Geometry check sheet. Reference: the model listing, model coordinates, mm. A direction names the side the tool comes from. Give positions to 0.01 mm unless a question says otherwise; leave off trailing zeros. Loops run counter-clockwise (first coordinate to the right, second up) from the corner with the lowest first, then second, coordinate; pieces in that order, holes last. Notation, with made-up numbers: (77, 43.25) -> (120, 43.25) arc R16 ccw to (120, 47.25) -> close; hole circle Ø2 at (5, 39). An arc over 180 degrees is marked (long way). One line per question, with ' | ' between items.
from build123d import *

# Parameters (mm, degrees)
IZIM1_R                     = 30
Y_KSEKLIK_EKSTR_ZYON1_DEPTH = 50
SCALE1_SCALE                = 0.5
SKETCH2_R                   = 12.5
CUT_EXTRUDE1_DEPTH          = 5
CUT_EXTRUDE2_START          = -10
SKETCH3_R                   = 12.5
CUT_EXTRUDE2_DEPTH          = 10
SKETCH4_R                   = 1
CUT_EXTRUDE3_DEPTH          = 10


with BuildPart() as part:
    # Çizim1 → Yükseklik-Ekstrüzyon1 (new body)
    with BuildSketch(Plane.XY):
        with Locations((-8.148787303, -1.554097453)):
            Circle(IZIM1_R)
    extrude(amount=Y_KSEKLIK_EKSTR_ZYON1_DEPTH)


with BuildPart() as part_1:
    # Scale1: scaled about (-8.148787303, -1.554097453, 25)
    add(part.part.scale(SCALE1_SCALE).moved(Location((-4.074393652, -0.777048727, 12.5))))

    # Sketch2 → Cut-Extrude1 (cut)
    with BuildSketch(Plane(origin=(0, 0, 12.5), x_dir=(-1, 0, 0), z_dir=(0, 0, -1))):
        with Locations((8.148787303, -1.554097453)):
            Circle(SKETCH2_R)
    extrude(amount=-CUT_EXTRUDE1_DEPTH, mode=Mode.SUBTRACT)

    # Sketch3 → Cut-Extrude2 (cut)
    with BuildSketch(Plane.XY.offset(37.5).offset(CUT_EXTRUDE2_START)):
        with Locations(Location((-8.148787303, -1.554097453, 0), (0, 0, 180))):
            Circle(SKETCH3_R)
    extrude(amount=CUT_EXTRUDE2_DEPTH, mode=Mode.SUBTRACT)

    # Sketch4 → Cut-Extrude3 (cut)
    with BuildSketch(Plane(origin=(0, 0, 17.5), x_dir=(-1, 0, 0), z_dir=(0, 0, -1))):
        with Locations((15.566518124, -5.706210793)):
            Circle(SKETCH4_R)
        with Locations((0.84408626, -5.901984113)):
            Circle(SKETCH4_R)
        with Locations((8.035757524, 6.945902547)):
            Circle(SKETCH4_R)
    extrude(amount=-CUT_EXTRUDE3_DEPTH, mode=Mode.SUBTRACT)


solid = part_1.part
Item 1: Scan lines: probe 1 along Z at (x, y) = (-6.75, -13.25); probe 2 along X at (y, z) = (-4.25, 30.75); probe 3 along Y at (x, z) = (-18, 30). Record each from-to range of solid material in increasing order.
Result:
probe 1: 17.5 to 27.5 | probe 2: -22.9 to -20.35, 4.06 to 6.61 | probe 3: -12.87 to -9.25, 6.14 to 9.76
Item 2: Sectioned sample at B-B (x = -15.25). Record the cut outline in (y, z), plus the area to 3 significant figures.
Result:
outline: (-14.77, 12.5) -> (-11.84, 12.5) -> (-11.84, 17.5) -> (-6.65, 17.5) -> (-6.65, 27.5) -> (-11.84, 27.5) -> (-11.84, 37.5) -> (-14.77, 37.5) -> close; (-4.76, 17.5) -> (8.73, 17.5) -> (8.73, 12.5) -> (11.66, 12.5) -> (11.66, 37.5) -> (8.73, 37.5) -> (8.73, 27.5) -> (-4.76, 27.5) -> close | area: 333 mm2
Item 3: Sectioned sample at D-D (y = -13.5). Record the cut outline in (x, z), plus the area to 3 significant figures.
Result:
outline: (-17.22, 12.5) -> (-11.83, 12.5) -> (-11.83, 17.5) -> (-4.47, 17.5) -> (-4.47, 12.5) -> (0.92, 12.5) -> (0.92, 37.5) -> (-4.47, 37.5) -> (-4.47, 27.5) -> (-11.83, 27.5) -> (-11.83, 37.5) -> (-17.22, 37.5) -> close | area: 343 mm2
Item 4: Sectioned sample at A-A (y = 7.5). Record the cut outline in (x, z), plus the area to 3 significant figures.
Result:
outline: (-20.11, 12.5) -> (-16.77, 12.5) -> (-16.77, 17.5) -> (-8.87, 17.5) -> (-8.87, 27.5) -> (-16.77, 27.5) -> (-16.77, 37.5) -> (-20.11, 37.5) -> close; (-7.2, 17.5) -> (0.47, 17.5) -> (0.47, 12.5) -> (3.81, 12.5) -> (3.81, 37.5) -> (0.47, 37.5) -> (0.47, 27.5) -> (-7.2, 27.5) -> close | area: 323 mm2
Item 5: Depth check by flat-ended pin: pin 1 Ø1.5 at (x, z) = (-17, 22) entering from +Y; pin 2 Ø3 at (y, z) = (9, 25) entering from +X; pin 3 Ø1 at (x, z) = (-7.5, 28.5) entering from -Y; pin 4 Ø2.5 at (x, y) = (-8.04, 6.95) entering from +Z. Enter the tip coordinate at first touch or a pass-through.
Result:
pin 1: y = 11.07 | pin 2: x = 3.81 | pin 3: y = -16.55 | pin 4: z = 27.5
Item 6: Release check for a two-part mould opening along Y. For faces 1 (the face through (-14, 10, 37.5)), 2 (the face through (-11.4, -16.197, 24.825)), 3 (the face through (0.155, -5.858, 22.43)) record: pulls with the +Y half, pulls with the -Y half, needs draft (parallel to the pull), parting line crosses it, or undercut.
Result:
face 1: needs draft | face 2: parting line crosses it | face 3: undercut
Item 7: Set-up check for faces 4 (the face through (-8, -2, 27.5)), 5 (the face through (-8, -1, 17.5)), 6 (the face through (-8.5, 6.06, 22.43)): record each of +Z, -Z, +X, -X, +Y, -Y from which the full face is reachable in a straight line by a thin tool's end or side.
Result:
face 4: +Z | face 5: -Z | face 6: +Z, -Z
Item 8: Sectioned sample at C-C (x = -6.5). Record the cut outline in (y, z), plus the area to 3 significant figures.
Result:
outline: (-16.46, 12.5) -> (-13.94, 12.5) -> (-13.94, 17.5) -> (10.84, 17.5) -> (10.84, 12.5) -> (13.36, 12.5) -> (13.36, 37.5) -> (10.84, 37.5) -> (10.84, 27.5) -> (-13.94, 27.5) -> (-13.94, 37.5) -> (-16.46, 37.5) -> close | area: 374 mm2
